Check sheet for the drawn part. Datum: minimum x, y, z corner. Units: mm. A direction names the side the tool comes from. Round coordinates to 2 decimals unless told otherwise and drop trailing zeros. Write each loop counter-clockwise with the first axis right and the second up, starting at its lowest first coordinate (ties: lowest second). Pieces come first, ordered by that corner, then holes. Notation, with made-up numbers: M -18.5,35 L 31.5,35 A10 ccw 31.5,50 Z; hole C 48,35 d7. An arc over 180 degrees is marked long. Put each result on its own line as item: value.
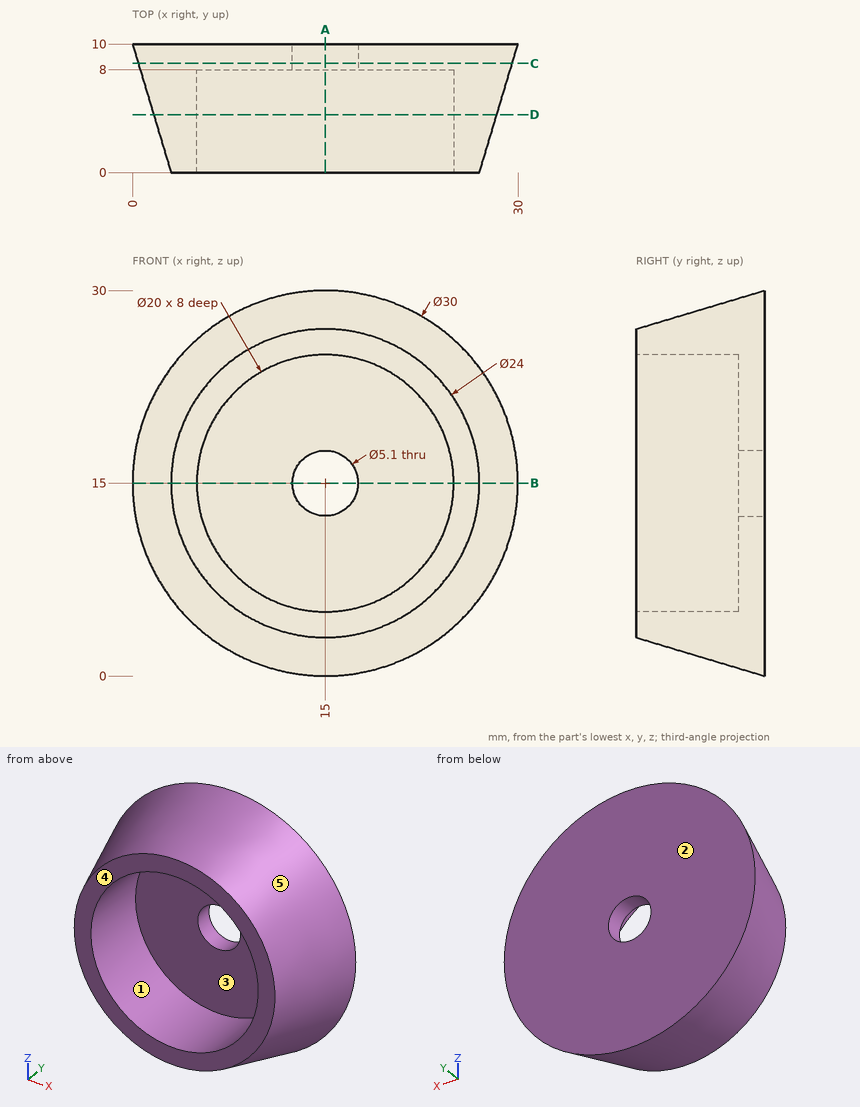
1. Scan lines: probe 1 along Y at (x, z) = (8.5, 16); probe 2 along Z at (x, y) = (9.5, 4.25); probe 3 along Z at (x, y) = (9, 4.25). Record each from-to range of solid material in increasing order.
Computed values:
probe 1: y = 8 to 10
probe 2: z = 2.92 to 6.65, 23.35 to 27.08
probe 3: z = 3.16 to 7, 23 to 26.84
2. Cross-section at A-A (x = 15). Enter the section's corners in (y, z), then the cut area to 3 significant figures.
Computed values:
outline: M 0,3 L 10,0 L 10,12.45 L 8,12.45 L 8,5 L 0,5 Z; M 0,25 L 8,25 L 8,17.55 L 10,17.55 L 10,30 L 0,27 Z
area: 99.8 mm2
3. Depth check by flat-ended pin: pin 1 Ø6.5 at (x, z) = (15, 15) entering from -Y; pin 2 Ø2 at (y, z) = (1.5, 8.5) entering from -X. Enter the tip coordinate at first touch or a pass-through.
Computed values:
pin 1: stops at y = 8
pin 2: stops at x = 3.73
4. Cross-section at C-C (y = 8.5). Enter the section's corners in (x, z).
Computed values:
outline: C 15,15 d29.1; hole C 15,15 d5.1
5. Access from +Z, -Z, +X, -X, +Y, -Y to the whole of each face (thin tool, end or side, straight path). Record for the marked faces 1 and 2.
Computed values:
face 1: -Y
face 2: +Z, -Z, +X, -X, +Y
6. Cross-section at D-D (y = 4.5). Enter the section's corners in (x, z).
Computed values:
outline: C 15,15 d26.7; hole C 15,15 d20
7. Release check for a two-part mould opening along Z. For the marked faces 3, 4 and 5 record: +Z half, -Z half, draft (parallel to the pull), parting line (faces both ways), or undercut.
Computed values:
face 3: undercut
face 4: draft
face 5: parting line
8. Cross-section at B-B (z = 15). Enter the section's corners in (x, y).
Computed values:
outline: M 0,10 L 3,0 L 5,0 L 5,8 L 12.45,8 L 12.45,10 Z; M 17.55,8 L 25,8 L 25,0 L 27,0 L 30,10 L 17.55,10 Z
